Source: CAD feature listing. Evaluate the final solid. Frame: model axes, mm. Face numbers are marked on the shaded views. A direction names the side the tool comes from. Round coordinates to 2 decimals unless told otherwise and drop trailing zeros. Order: outer loops, then holes, each group sorted by start corner. A loop starts at its lowest first (then second) coordinate and runs counter-clockwise, first axis right, second up. Notation, with made-up numbers: M 85,46.25 L 93,46.25 A25 cw 93,73.25 Z; hole C 35.25,31 d2. An arc over 180 degrees is marked long. Answer as CSV lines item,"result". Start each with the question number.
Item 1: First-contact query: P1, Ø1, axis at x = 3, y = -2, coming from the -Z side; P2, Ø5, axis at y = -7, z = 6, coming from the +X side; P3, Ø2, axis at x = 17, z = 0.5, coming from the +Y side. Flat tips, straight axial feed; report the tip coordinate or a pass-through.
Item 2: Section query A-A on x = 17. Return the cut outline in (y, z), plus the area to 3 significant figures.
Item 3: Set-up query: the marked faces 1 and 2. Return all of +Z, -Z, +X, -X, +Y, -Y with unobstructed straight access to the full face (end or side cutting, diameter ignored); none if empty.
Item 4: Line query: line 1 (Y direction, x = 6.5, z = 0); line 2 (X direction, y = -4, z = 6). Output: solid intervals per line, ascending. Write a range as [from, to].
Autodesk Inventor part; units mm, degrees
ref_plane "Work Plane1" through (1.525, 0, 0) normal (0, 0, 1) x (1, 0, 0)
ref_plane "YZ Plane" through (0, 0, 0) normal (1, 0, 0) x (0, 1, 0)
ref_plane "XZ Plane" through (0, 0, 0) normal (0, 1, 0) x (-1, 0, 0)
sketch "Sketch1" plane through (0, 0, 0) normal (0, 0, 1) x (1, 0, 0)
  line L0 (0, 7.315) -> (0, 5)
  line L1 (3, 5) -> (20, 5)
  line L2 (20, 5) -> (20, 0)
  line L3 (20, 0) -> (-0.6001, 0)
  line L4 (-4.7201, 0) -> (24.12, 0)
  line L5 (-0.6001, 0) -> (-0.6001, 7.315)
  line L6 (-0.6001, 7.315) -> (0, 7.315)
  line L7 (3, 5) -> (2.3865, 5)
  line L8 (2.3865, 5) -> (0, 5)
  line L9 (0, -1.463) -> (0, 8.778)
  dimension "d0" = 20
  dimension "d1" = 17
  dimension "d2" = 10
  dimension "d9" = 0.6001
  dimension "d10" = 14.63
  dimension "d13" = 0.6136
  dimension "d14" = 10
revolve "Body" add sketch "Sketch1" angle 360 about axis through (20, 0, 0) along (-1, 0, 0)
sketch "Sketch2" plane through (-0.6001, 0, 0) normal (-1, 0, 0) x (0, 0, 1)
  line L0 (0, 9.2376) -> (8, 4.6188)
  line L1 (8, 4.6188) -> (8, -4.6188)
  line L2 (8, -4.6188) -> (0, -9.2376)
  line L3 (0, -9.2376) -> (-8, -4.6188)
  line L4 (-8, -4.6188) -> (-8, 4.6188)
  line L5 (-8, 4.6188) -> (0, 9.2376)
  point P0 (0, 0)
  point P1 (0, 0)
  dimension "d11" = 16
extrude "Head" add sketch "Sketch2" along normal blind 5.8
sketch "Sketch4" plane through (0, 0, 0) normal (0, 0, 1) x (1, 0, 0)
  line L0 (-6.4001, 8) -> (-6.4001, 9.2376)
  line L1 (-6.4001, 9.2376) -> (-5.6856, 9.2376)
  line L2 (-5.6856, 9.2376) -> (-6.4001, 8)
  line L3 (-7.5601, 0) -> (0.5599, 0)
  line L4 (-0.6001, 9.2376) -> (-6.4001, 9.2376)
  line L5 (-6.4001, 4.6188) -> (-6.4001, 9.2376)
  dimension "d5" = 30
  dimension "d19" = 16
revolve "Chamfer1" cut sketch "Sketch4" angle 360 about axis through (-10, 0, 0) along (1, 0, 0)
thread "Thread"
chamfer "Chamfer2" distance 0.6134 distance2 0.6136 1 edges at (20, -5, 0) measured on face at (20, -0.8193, 0.3214)
ref_plane "Work Plane1" through (1.525, 0, 0) normal (0, 0, 1) x (1, 0, 0)
equation "\"d0\" = NLG"
equation "\"d1\" = GEL"
equation "\"d2\" = GD"
equation "\"d10\" = SD2"
equation "\"d14\" = BDM"
equation "\"d11\" = SW"
equation "\"d3\" = KOH - SD"
equation "\"d5\" = ANG1"
equation "\"d19\" = SW0"
equation "\"d15\" = GEL"
equation "\"d6\" = -0.5 * SPD + 0.5 * GD"
equation "\"NLG\" = 20"
equation "\"GD\" = NND"
equation "\"BDM\" = NND"
equation "\"KOH\" = 6.4"
equation "\"GEL\" = 17"
equation "\"SW\" = 16"
equation "\"SW0\" = 16"
equation "\"SPD\" = NND - 1.2269 * PTC"
equation "\"SD2\" = 14.63"
equation "\"SD\" = 0.6"
equation "\"ANG1\" = 30deg"
equation "\"GAL\" = 0.61345 * PTC"
equation "\"GUL\" = 0.61345 * PTC"
equation "\"RR\" = 0.4"
equation "\"GD1\" = THREADDIA - 1.2269 * PTC"
equation "\"SDH\" = SD2"
equation "\"TOA\" = 30deg"
equation "\"PTC\" = 1"
equation "\"E0\" = 1.155 * SW"
properties part number "ISO 8676 - M10 x 1 x 20" material "Stainless Steel, 440C"
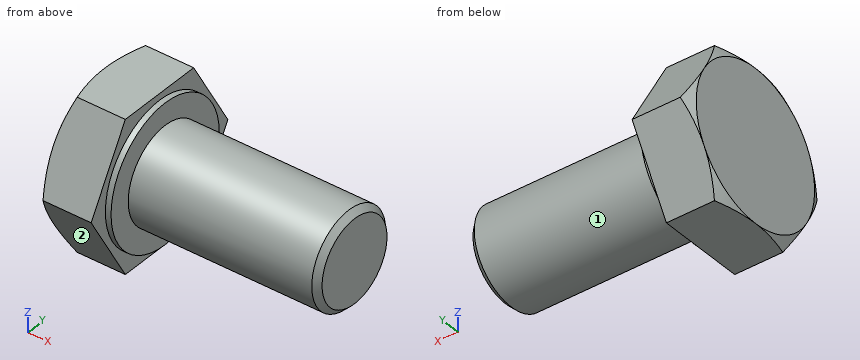
Results:
1,P1,"z = -4.77"
1,P2,"x = 0"
1,P3,"y = 5"
2,outline,"C 0,0 d10"
2,area,"78.5 mm^2"
3,face 1,"+X"
3,face 2,"-Z, +X, -X, -Y"
4,line 1,"[-5, 5]"
4,line 2,"[-6.4, 0]"
